from build123d import *

# Parameters (mm, degrees)
BOSS_EXTRUDE1_DEPTH     = 29
CUT_EXTRUDE1_DEPTH      = 39.173943993
CUT_EXTRUDE1_DEPTH_BACK = 39.173943993
SKETCH2_R               = 2.575
FILLET1_R               = 4.5
FILLET2_R               = 4
CHAMFER1_SIZE           = 0.25
CHAMFER1_SIZE2          = 0.686869355
FILLET4_R               = 0.25


with BuildPart() as part:
    # Sketch1 → Boss-Extrude1 (new body)
    with BuildSketch(Plane(origin=(0, 0, 0), x_dir=(1, 0, 0), z_dir=(0, 1, 0))):
        Polygon((0, 0), (0, 3.8), (8.5, 3.8), (12.5, 7.8), (20.5, 7.8), (24.5, 3.8), (24.5, 2.25), (22.5, 2.25), (22.5, 2.971572875), (19.671572875, 5.8), (13.328427125, 5.8), (9, 1.471572875), (9, 0), align=None)
    extrude(amount=BOSS_EXTRUDE1_DEPTH)

    # Sketch2 → Cut-Extrude1 (cut, two sides: drawn at the far end of the back side and taken through both)
    with BuildSketch(Plane(origin=(0, 0, -3.8), x_dir=(-1, 0, 0), z_dir=(0, 0, -1)).offset(-CUT_EXTRUDE1_DEPTH_BACK)):
        with Locations((-4.25, 4.5)):
            Circle(SKETCH2_R)
        with Locations((-4.25, 24.5)):
            Circle(SKETCH2_R)
    extrude(amount=CUT_EXTRUDE1_DEPTH + CUT_EXTRUDE1_DEPTH_BACK, mode=Mode.SUBTRACT)

    # Fillet1
    fillet1_edges = [part.edges().sort_by_distance(p)[0] for p in [
        (0, 0, -1.9),
        (0, 29, -1.9),
    ]]
    fillet(fillet1_edges, radius=FILLET1_R)

    # Fillet2
    # the kernel refuses this fillet: 4 mm, written as the material it adds along each edge
    with BuildSketch(Plane(origin=(9, 0, -1.471572875), x_dir=(0, 0, 1), z_dir=(0, 1, 0))) as fillet2_piece_1:
        with BuildLine():
            CenterArc((1.66135914, 3.99549511), FILLET2_R, 225, 42.280491011)
            Line((-1.167067985, 1.167067985), (-1.223636528, 1.110499443))
            Line((-1.223636528, 1.110499443), (-0.056568542, -0.056568542))
            Line((-0.056568542, -0.056568542), (0, -0.08))
            ThreePointArc((0, -0.08), (0.735786438, -0.08), (1.46777715, -0.079909902))
            Line((1.46777715, -0.079909902), (1.471572875, 0))
        make_face()
    extrude(amount=29)
    with BuildSketch(Plane(origin=(19.671572875, 0, -5.8), x_dir=(-1, 0, 0), z_dir=(0, 1, 0)), Plane(origin=(13.328427125, 0, -5.8), x_dir=(-0.7071067811865457, 0, 0.7071067811865493), z_dir=(0, 1, 0))) as fillet2_piece_2:
        with BuildLine():
            CenterArc((FILLET2_R * 0.414213562373, FILLET2_R), FILLET2_R, 225, 45)
            Line((-FILLET2_R * 0.292893218813, FILLET2_R * 0.292893218813), (-FILLET2_R * 0.307035354437, FILLET2_R * 0.27875108319))
            Line((-FILLET2_R * 0.307035354437, FILLET2_R * 0.27875108319), (-FILLET2_R * 0.00828427124746, -FILLET2_R * 0.02))
            Line((-FILLET2_R * 0.00828427124746, -FILLET2_R * 0.02), (FILLET2_R * 0.414213562373, -FILLET2_R * 0.02))
            Line((FILLET2_R * 0.414213562373, -FILLET2_R * 0.02), (FILLET2_R * 0.414213562373, 0))
        make_face()
    extrude(amount=29)
    with BuildSketch(Plane(origin=(22.5, 0, -2.971572875), x_dir=(-0.7071067811865455, 0, -0.7071067811865495), z_dir=(0, 1, 0))) as fillet2_piece_3:
        with BuildLine():
            CenterArc((1.444636364, 4), FILLET2_R, 240.743753532, 29.256246468)
            Line((-0.510229073, 0.510229073), (-0.549326382, 0.440433655))
            ThreePointArc((-0.549326382, 0.440433655), (-0.311683079, 0.198545994), (-0.056568542, -0.056568542))
            Line((-0.056568542, -0.056568542), (0, -0.08))
            Line((0, -0.08), (1.444636364, -0.08))
            Line((1.444636364, -0.08), (1.444636364, 0))
        make_face()
    extrude(amount=29)
    # the kernel refuses this fillet: 4 mm, written as the material it takes off along each edge
    with BuildSketch(Plane(origin=(20.5, -4.142135624, -7.8), x_dir=(0.7071067811865446, 0, 0.7071067811865505), z_dir=(0, 1, 0))) as fillet2_2_piece_1:
        with BuildLine():
            CenterArc((FILLET2_R * 0.414213562373, -FILLET2_R), FILLET2_R, 90, 45)
            Line((-FILLET2_R * 0.292893218813, -FILLET2_R * 0.292893218813), (-FILLET2_R * 0.307035354437, -FILLET2_R * 0.27875108319))
            Line((-FILLET2_R * 0.307035354437, -FILLET2_R * 0.27875108319), (-FILLET2_R * 0.00828427124746, FILLET2_R * 0.02))
            Line((-FILLET2_R * 0.00828427124746, FILLET2_R * 0.02), (FILLET2_R * 0.414213562373, FILLET2_R * 0.02))
            Line((FILLET2_R * 0.414213562373, FILLET2_R * 0.02), (FILLET2_R * 0.414213562373, 0))
        make_face()
    extrude(amount=37.284271247, mode=Mode.SUBTRACT)
    with BuildSketch(Plane(origin=(12.5, -4.142135624, -7.8), x_dir=(-0.7071067811865461, 0, 0.7071067811865489), z_dir=(0, 1, 0))) as fillet2_2_piece_2:
        with BuildLine():
            CenterArc((FILLET2_R * 0.414213562373, FILLET2_R), FILLET2_R, 225, 45)
            Line((-FILLET2_R * 0.292893218813, FILLET2_R * 0.292893218813), (-FILLET2_R * 0.307035354437, FILLET2_R * 0.27875108319))
            Line((-FILLET2_R * 0.307035354437, FILLET2_R * 0.27875108319), (-FILLET2_R * 0.00828427124746, -FILLET2_R * 0.02))
            Line((-FILLET2_R * 0.00828427124746, -FILLET2_R * 0.02), (FILLET2_R * 0.414213562373, -FILLET2_R * 0.02))
            Line((FILLET2_R * 0.414213562373, -FILLET2_R * 0.02), (FILLET2_R * 0.414213562373, 0))
        make_face()
    extrude(amount=37.284271247, mode=Mode.SUBTRACT)
    with BuildSketch(Plane(origin=(24.5, -4.136949157, -3.8), x_dir=(0, 0, 1), z_dir=(0, 1, 0))) as fillet2_2_piece_3:
        with BuildLine():
            CenterArc((1.658321204, -3.998533046), FILLET2_R, 91.551776657, 43.448223343)
            Line((-1.170105921, -1.170105921), (-1.226674463, -1.113537378))
            Line((-1.226674463, -1.113537378), (-0.056568542, 0.056568542))
            Line((-0.056568542, 0.056568542), (0, 0.08))
            ThreePointArc((0, 0.08), (0.775, 0.08), (1.547833576, 0.079970661))
            Line((1.547833576, 0.079970661), (1.55, 0))
        make_face()
    extrude(amount=37.273898313, mode=Mode.SUBTRACT)

    # Chamfer1
    chamfer1_edges = [part.edges().sort_by_distance(p)[0] for p in [
        (6.825, 4.5, 0),
        (6.825, 24.5, 0),
    ]]
    chamfer1_side = [part.faces().sort_by_distance(p)[0] for p in [
        (4.693643045, 14.5, 0),
    ]]
    chamfer(chamfer1_edges, length=CHAMFER1_SIZE, length2=CHAMFER1_SIZE2, reference=chamfer1_side[0])

    # Fillet4
    fillet4_edges = [part.edges().sort_by_distance(p)[0] for p in [
        (24.5, 14.5, -2.25),
        (22.5, 14.5, -2.25),
    ]]
    fillet(fillet4_edges, radius=FILLET4_R)


solid = part.part
Geometry: final body of the model. Coordinates: model frame, mm. A direction names the side the tool comes from. Give positions to 0.01 mm unless a question says otherwise; leave off trailing zeros. Write each loop counter-clockwise with the first axis right and the second up, starting at its lowest first coordinate (ties: lowest second). Pieces come first, ordered by that corner, then holes.
(1) Cut plane A-A, the plane z = -1.25. Return loops of the section in (x, y) (3 decimals), then the cut area to 3 significant figures.
(2) Cut plane C-C, the plane x = 3. Give the number of separate pieces and of enclosed holes in the cut face, then the cut area to 3 significant figures.
(3) Cut plane B-B, the plane y = 20.25. Return loops of the section in (x, z), then the cut area to 3 significant figures.
(4) Mould query, pull axis Y, two halves, no side actions, for faces 4 (the flat face through (12, 29, -5)), 5 (the cylindrical face through (3.062, 2.216, -2.222)), 6 (the cylindrical face through (22.062, 14.297, -3.253)). Classes: released by +Y, released by -Y, zero draft, split by the parting line, or undercut.
(5) Access query for faces 1 (the flat face through (4, 14, -3.8)), 2 (the flat face through (17, 14, -5.8)), 3 (the flat face through (23, 14, -2.25)). Directions: +Z, -Z, +X, -X, +Y, -Y. A direction counts if a zero-diameter tool reaches every point of the face in a straight line with its end or side. Return the directions, or none.
(6) First-contact query: P1, Ø4, axis at x = 12, y = 15.5, coming from the +Z side; P2, Ø7, axis at x = 5.5, y = 16, coming from the -Z side; P3, Ø1.2, axis at x = 23, y = 11.5, coming from the +Z side. Flat tips, straight axial feed; report the tip coordinate or a pass-through.
(7) Cut plane D-D, the plane x = 16.25. Return loops of the section in (y, z), then the cut area to 3 significant figures.
(8) Ray query, line 1 (Y direction, x = 4.25, z = -3.05) (3 decimals); line 2 (X direction, y = 5.25, z = -3.5); line 3 (X direction, y = 2.5, z = -3). Return the intervals inside material, ascending.
Values follow:
1. outline: (0, 4.5) arc R4.5 ccw to (4.5, 0) - (9.264, 0) - (9.264, 29) - (4.5, 29) arc R4.5 ccw to (0, 24.5) - close; hole circle Ø5.15 at (4.25, 4.5); hole circle Ø5.15 at (4.25, 24.5)
1. area: 218 mm2
2. separate pieces: 3
2. enclosed holes: 0
2. area: 73.6 mm2
3. outline: (0, -3.8) - (8.5, -3.8) - (11.33, -6.63) arc R4 ccw to (14.16, -7.8) - (18.84, -7.8) arc R4 ccw to (21.67, -6.63) - (23.33, -4.97) arc R4 ccw to (24.48, -2.52) arc R0.25 ccw to (24.23, -2.25) - (22.68, -2.25) arc R0.25 ccw to (22.45, -2.42) arc R4 cw to (21.48, -3.99) - (20.84, -4.63) arc R4 cw to (18.01, -5.8) - (14.99, -5.8) arc R4 cw to (12.16, -4.63) - (10.17, -2.64) arc R4 cw to (9, 0) - (0, 0) - close
3. area: 71.8 mm2
4. face 4: released by +Y
4. face 5: undercut
4. face 6: zero draft
5. face 1: -Z, -X, +Y, -Y
5. face 2: +Z, +Y, -Y
5. face 3: +Z, +X, +Y, -Y
6. P1: stops at z = -2.46
6. P2: stops at z = -4.3
6. P3: stops at z = -2.25
7. outline: (0, -7.8) - (29, -7.8) - (29, -5.8) - (0, -5.8) - close
7. area: 58.0 mm2
8. line 1: y = 0.007 to 1.925, 7.075 to 21.925, 27.075 to 28.993
8. line 2: x = 0 to 1.79, 6.71 to 11.03, 21.9 to 24.26
8. line 3: x = 0.47 to 2.63, 5.87 to 10.53, 22.2 to 24.41
